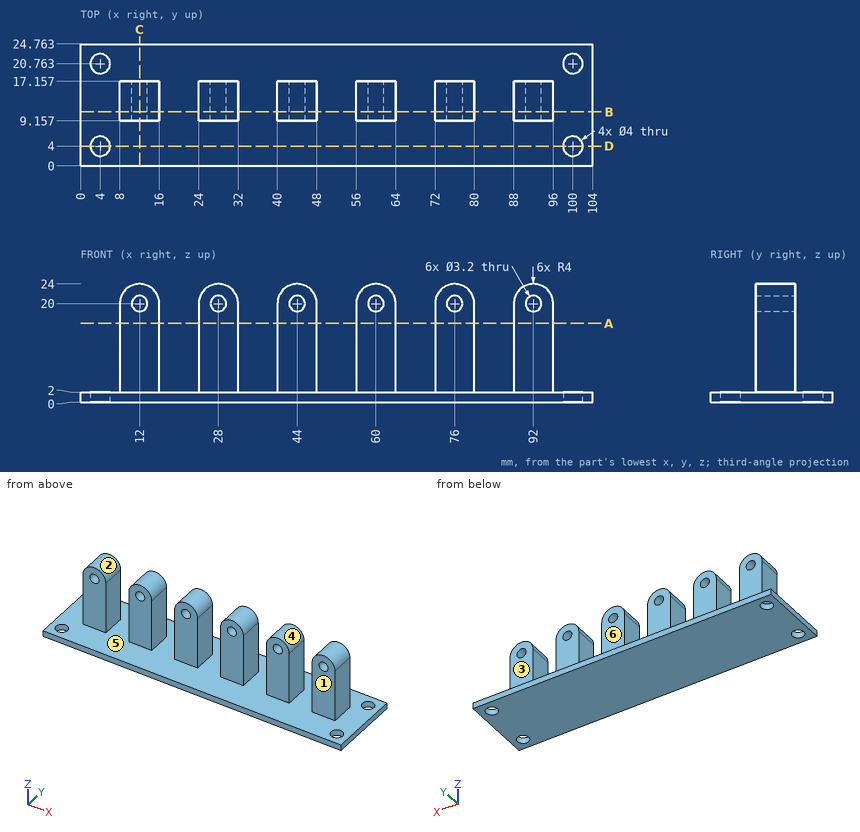
Check sheet for the drawn part. Datum: minimum x, y, z corner. Units: mm. A direction names the side the tool comes from. Round coordinates to 2 decimals unless told otherwise and drop trailing zeros. Order: outer loops, then holes, each group sorted by start corner. A loop starts at its lowest first (then second) coordinate and runs counter-clockwise, first axis right, second up. Notation, with made-up numbers: M 67,13 L 102,13 A15 ccw 102,18 Z; hole C 23,54.25 d3. An arc over 180 degrees is marked long. Write each question's results on one line, items separated by ' | '. Start each with the question number.
1. Draft check along X on the marked faces 4, 5 and 6. Enter one of: pulls with the +X half, pulls with the -X half, needs draft (parallel to the pull), parting line crosses it, or undercut.
2. Go/stop test with flat-tipped pins: P1, Ø4, axis at x = 60, z = 20, coming from the +Y side; P2, Ø6.5, axis at x = 91, z = 17.5, coming from the -Y side; P3, Ø2.5, axis at y = 13.5, z = 14.5, coming from the +X side; P4, Ø4, axis at y = 6, z = 17.5, coming from the +X side (3 decimals). Record where each tip stops, or that it passes through.
3. Cross-section at A-A on z = 16. Record the boundary of the cut face in (x, y), plus the area to 3 significant figures.
4. Cross-section at D-D on y = 4. Record the boundary of the cut face in (x, z), plus the area to 3 significant figures.
5. Cross-section at B-B on y = 11. Give the number of separate pieces and of enclosed holes in the cut face, plus the area to 3 significant figures.
6. Material ranges on L1, parallel to X at y = 15, z = 16.75; L2, parallel to Y at x = 4, z = 1.2; L3, parallel to Z at x = 28, y = 14.5, recorded low to high. Write a range as from..to.
7. Cross-section at C-C on x = 12. Record the boundary of the cut face in (y, z), plus the area to 3 significant figures.
8. Set-up check for the marked faces 1, 2 and 3: record each of +Z, -Z, +X, -X, +Y, -Y from which the full face is reachable in a straight line by a thin tool's end or side.
Resolved:
1) face 4: undercut | face 5: undercut | face 6: needs draft
2) P1: y = 17.16 | P2: y = 9.16 | P3: x = 96 | P4: through
3) outline: M 8,9.16 L 16,9.16 L 16,17.16 L 8,17.16 Z; M 24,9.16 L 32,9.16 L 32,17.16 L 24,17.16 Z; M 40,9.16 L 48,9.16 L 48,17.16 L 40,17.16 Z; M 56,9.16 L 64,9.16 L 64,17.16 L 56,17.16 Z; M 72,9.16 L 80,9.16 L 80,17.16 L 72,17.16 Z; M 88,9.16 L 96,9.16 L 96,17.16 L 88,17.16 Z | area: 384 mm2
4) outline: M 0,0 L 2,0 L 2,2 L 0,2 Z; M 6,0 L 98,0 L 98,2 L 6,2 Z; M 102,0 L 104,0 L 104,2 L 102,2 Z | area: 192 mm2
5) separate pieces: 1 | enclosed holes: 6 | area: 1,170 mm2
6) L1: 8..16, 24..32, 40..48, 56..64, 72..80, 88..96 | L2: 0..2, 6..18.76, 22.76..24.76 | L3: 0..18.4, 21.6..24
7) outline: M 0,0 L 24.76,0 L 24.76,2 L 17.16,2 L 17.16,18.4 L 9.16,18.4 L 9.16,2 L 0,2 Z; M 9.16,21.6 L 17.16,21.6 L 17.16,24 L 9.16,24 Z | area: 200 mm2
8) face 1: +Z, +X, -X, -Y | face 2: +Z, +Y, -Y | face 3: +Z, +X, -X, +Y
